The model under review builds one solid part; all positions refer to its coordinate system, in mm. Face numbers are marked on the shaded views. A direction names the side the tool comes from. Coordinates: 2 decimals unless noted, no trailing zeros. Loops run counter-clockwise (first coordinate to the right, second up) from the corner with the lowest first, then second, coordinate; pieces in that order, holes last. Notation, with made-up numbers: M 66.25,-23 L 95.25,-23 A12 cw 95.25,-11 Z; hole C -27.75,38.5 d5. An arc over 180 degrees is marked long. Use one line per item in the form item = value.
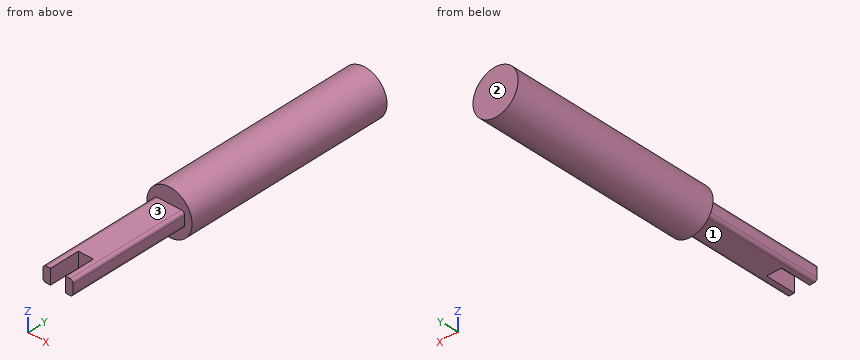
```python
from build123d import *

# Parameters (mm, degrees)
F0_R     = 9.525
F1_DEPTH = 88.9
F2_W     = 12.7
F2_H     = 6.35
F3_DEPTH = 50.8
F4_W     = 6.35
F4_H     = 6.35
F5_DEPTH = 12.7
F6_R     = 1.27


with BuildPart() as f1:
    # F0 (on Front) → F1 (new body)
    with BuildSketch(Plane.XZ):
        Circle(F0_R)
    extrude(amount=-F1_DEPTH)

    # F2 (on face) → F3 (join)
    with BuildSketch(Plane.XZ):
        Rectangle(F2_W, F2_H)
    extrude(amount=F3_DEPTH)

    # F4 (on face) → F5 (cut)
    with BuildSketch(Plane.XZ.offset(50.8)):
        Rectangle(F4_W, F4_H)
    extrude(amount=-F5_DEPTH, mode=Mode.SUBTRACT)

    # F6
    f6_edges = [f1.edges().sort_by_distance(p)[0] for p in [
        (6.35, -25.4, 3.175),
        (-6.35, -25.4, 3.175),
        (-6.35, -25.4, -3.175),
        (6.35, -25.4, -3.175),
    ]]
    fillet(f6_edges, radius=F6_R)


solid = f1.part
```
1. Add section B-B (y = -25). State the section outline as (x, z) points (3 decimals).
Response values:
outline = M -6.35,-1.905 A1.27 ccw -5.08,-3.175 L 5.08,-3.175 A1.27 ccw 6.35,-1.905 L 6.35,1.905 A1.27 ccw 5.08,3.175 L -5.08,3.175 A1.27 ccw -6.35,1.905 Z
2. Insertion check: P1, Ø1.1, axis at y = -13.5, z = 0.5, coming from the -X side; P2, Ø5, axis at y = -42.5, z = -1, coming from the +X side; P3, Ø6, axis at x = 6, y = 38.5, coming from the -Z side. Each pin has a flat end and moves straight along its axis. Give the tip position at first contact, or say it passes through.
Response values:
P1 = -6.35
P2 = 6.35
P3 = -9.04
3. Machinability: for the marked faces 1, 2 and 3, which of the approach directions +Z, -Z, +X, -X, +Y, -Y give a long, thin tool a straight path to every point of the face, cutting with its end or side? Answer none if there is none.
Response values:
face_1 = -Z, +X, -X, -Y
face_2 = +Z, -Z, +X, -X, +Y
face_3 = +Z, +X, -X, -Y
4. Wall thickness on line 1 along X through (y, z) = (66.5, -0.25); line 2 along Y through (x, z) = (0.5, 8.25); line 3 along Z through (x, y) = (-4.75, -11.5) (3 decimals): over which ranges is each line inside the solid? List them lowest first. Write a range as from..to.
Response values:
line_1 = -9.52..9.52
line_2 = 0..88.9
line_3 = -3.175..3.175
5. Add section D-D (y = 5). State the section outline as (x, z) points (3 decimals).
Response values:
outline = C 0,0 d19.05
6. Add section A-A (x = 0). State the section outline as (y, z) points (3 decimals).
Response values:
outline = M -38.1,-3.175 L 0,-3.175 L 0,-9.525 L 88.9,-9.525 L 88.9,9.525 L 0,9.525 L 0,3.175 L -38.1,3.175 Z
7. Add section C-C (z = 0). State the section outline as (x, y) points (3 decimals).
Response values:
outline = M -9.525,0 L -6.35,0 L -6.35,-50.8 L -3.175,-50.8 L -3.175,-38.1 L 3.175,-38.1 L 3.175,-50.8 L 6.35,-50.8 L 6.35,0 L 9.525,0 L 9.525,88.9 L -9.525,88.9 Z
